Model file for the job. Use its own axes, mm. A direction names the side the tool comes from. Coordinates: 2 decimals unless noted, no trailing zeros. Write each loop counter-clockwise with the first axis right and the second up, starting at its lowest first coordinate (ties: lowest second). Pieces come first, ordered by that corner, then holes. Notation, with made-up numbers: (87, 75) -> (129, 75) arc R18 cw to (129, 82) -> close; hole circle Ø11 at (-24, 79.25). An arc over 180 degrees is marked (long way). Answer as a JSON object with one key per item and string values. Group by question number.
Autodesk Inventor part; units mm, degrees
ref_plane "YZ Plane" through (0, 0, 0) normal (1, 0, 0) x (0, 1, 0)
ref_plane "XZ Plane" through (0, 0, 0) normal (0, 1, 0) x (-1, 0, 0)
ref_plane "XY Plane" through (0, 0, 0) normal (0, 0, 1) x (1, 0, 0)
sketch "草图1" plane through (0, 0, 0) normal (0, 0, 1) x (1, 0, 0)
  circle A0 centre (0, 0) radius 225
  dimension "d0" = 450
surface extrude "拉伸曲面1" sketch "草图1" along normal blind 200 shown no curves A0
thicken "加厚1" operation new thickness 3.7 both sides no extend neighbours no toward (-0.4864037, 0.8737342, 0) faces at (109.4408, -196.5902, 133.3333)
sketch "草图2" plane through (0, 0, 200) normal (0, 0, 1) x (1, 0, 0)
  circle A0 centre (0, 0) radius 225
  circle A1 centre (0, 0) radius 221.3
  circle A2 centre (0, 0) radius 290
  dimension "d18" = 580
  dimension "d19" = 442.6
  dimension "d20" = 450
extrude "拉伸1" add sketch "草图2" against normal blind 15 contours A2
sketch "草图3" plane through (0, 0, 200) normal (0, 0, 1) x (1, 0, 0)
  circle A0 centre (0, 0) radius 290
  circle A1 centre (0, 0) radius 221.3
  line L0 (0, -221.3) -> (0, -290)
  point P0 (0, -255.65)
  point P1 (180.7718, -180.7718)
  point P2 (255.65, 0)
  point P3 (180.7718, 180.7718)
  point P4 (0, 255.65)
  point P5 (-180.7718, 180.7718)
  point P6 (-255.65, 0)
  point P7 (-180.7718, -180.7718)
  dimension "d9" = 360
  dimension "d21" = 255.65
hole "孔1" at (0, -255.65, 200) at (180.7718, -180.7718, 200) at (255.65, 0, 200) at (180.7718, 180.7718, 200) at (0, 255.65, 200) at (-180.7718, 180.7718, 200) at (-255.65, 0, 200) at (-180.7718, -180.7718, 200) direction (0, 0, -1) diameter 20 end through all
sketch "草图4" plane through (0, 0, 0) normal (1, 0, 0) x (0, 1, 0)
  line L0 (-225, 185) -> (225, 185)
  line L1 (225, 0) -> (-225, 0)
  line L2 (225, 0) -> (-225, 0)
  line L3 (-225, 0) -> (225, 92.5)
  line L4 (225, 0) -> (225, 185)
  point P0 (0, 0)
extrude "拉伸2" [suppressed]
properties part number "人孔"
(1) Cut at C-C on y = -143.5. List the corners of the cut face in (x, z), plus the area to 3 significant figures.
(2) Pull direction Y, two halves, no side cores. Call faces 1 (the face through (-189.204, -186.148, 192.395)), 2 (the face through (276.608, 87.108, 192.605)), 3 (the face through (180.332, 190.762, 192.395)), 4 (the face through (-216, 66, 185)): released by +Y, released by -Y, zero draft, split by the parting line, or undercut.
(3) Cut at A-A on y = 0. List the corners of the cut face in (x, z), plus the area to 3 significant figures.
(4) Wall check: probe 1 along Y at (x, z) = (0, 196); probe 2 along Y at (x, z) = (2, 85.5); probe 3 along X at (y, z) = (-193, 41). Give the ranges that are in metal, low to high.
(5) Pin check, flat tips, straight feed: pin 1 (18 mm diameter, centred on x = -255.65, y = 0, fed in from +Z); pin 2 (12 mm diameter, centred on y = 176.5, z = 134, fed in from +X); pin 3 (2 mm diameter, centred on y = 50.5, z = 82.5, fed in from +X); pin 4 (8 mm diameter, centred on x = 199, z = 86.5, fed in from +Y). Stop position of each tip, or through.
(6) 3-axis set-ups, long thin cutter, end or side, ignore diameter. For faces 5 (the face through (-224.782, -9.893, 91.205)), 6 (the face through (184.6, -190.01, 192.4)): which of +Z, -Z, +X, -X, +Y, -Y reach the whole face in a straight line?
(7) Cut at D-D on x = -214.5. List the corners of the cut face in (y, z), plus the area to 3 significant figures.
Results found:
{
 "1": {"outline": "(-252.01, 185) -> (-173.3, 185) -> (-173.3, 0) -> (-168.47, 0) -> (-168.47, 200) -> (-252.01, 200) -> close; (168.47, 0) -> (173.3, 0) -> (173.3, 185) -> (252.01, 185) -> (252.01, 200) -> (168.47, 200) -> close", "area": "4,290 mm²"},
 "2": {"face 1": "undercut", "face 2": "split by the parting line", "face 3": "undercut", "face 4": "zero draft"},
 "3": {"outline": "(-290, 185) -> (-265.65, 185) -> (-265.65, 200) -> (-290, 200) -> close; (-245.65, 185) -> (-225, 185) -> (-225, 0) -> (-221.3, 0) -> (-221.3, 200) -> (-245.65, 200) -> close; (221.3, 0) -> (225, 0) -> (225, 185) -> (245.65, 185) -> (245.65, 200) -> (221.3, 200) -> close; (265.65, 185) -> (290, 185) -> (290, 200) -> (265.65, 200) -> close", "area": "2,830 mm²"},
 "4": {"probe 1": "y = -290 to -265.65, -245.65 to -221.3, 221.3 to 245.65, 265.65 to 290", "probe 2": "y = -224.99 to -221.29, 221.29 to 224.99", "probe 3": "x = -115.65 to -108.28, 108.28 to 115.65"},
 "5": {"pin 1": "passes through", "pin 2": "stops at x = 146.82", "pin 3": "stops at x = 219.49", "pin 4": "stops at y = 112.25"},
 "6": {"face 5": "-Z", "face 6": "+Z, -Z"},
 "7": {"outline": "(-195.17, 185) -> (-67.93, 185) -> (-67.93, 0) -> (-54.44, 0) -> (-54.44, 200) -> (-195.17, 200) -> close; (54.44, 0) -> (67.93, 0) -> (67.93, 185) -> (195.17, 185) -> (195.17, 200) -> (54.44, 200) -> close", "area": "9,210 mm²"}
}
